Part model, mm, in its own coordinate system. Face numbers are marked on the shaded views. A direction names the side the tool comes from. Coordinates: 2 decimals unless noted, no trailing zeros. Order: outer loops, then holes, each group sorted by start corner. A loop starts at its lowest first (then second) coordinate and runs counter-clockwise, first axis right, second up.
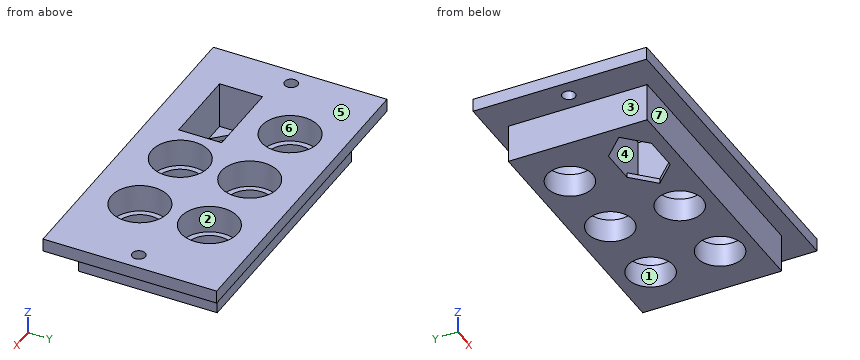
Autodesk Inventor part; units mm, degrees
ref_plane "YZ Plane" through (0, 0, 0) normal (1, 0, 0) x (0, 1, 0)
ref_plane "XZ Plane" through (0, 0, 0) normal (0, 1, 0) x (-1, 0, 0)
ref_plane "XY Plane" through (0, 0, 0) normal (0, 0, 1) x (1, 0, 0)
sketch "Sketch1" plane through (0, 0, 0) normal (0, 0, 1) x (1, 0, 0)
  line L0 (0, 0) -> (47.625, 0)
  line L1 (47.625, 0) -> (47.625, 25.4)
  line L2 (47.625, 25.4) -> (0, 25.4)
  line L3 (0, 25.4) -> (0, 0)
  circle A0 centre (38.1, 6.35) radius 5.207
  circle A1 centre (23.8125, 6.35) radius 5.207
  circle A2 centre (23.8125, 19.05) radius 5.207
  circle A3 centre (38.1, 19.05) radius 5.207
  circle A4 centre (9.525, 19.05) radius 5.207
  line L4 (2.2603, 10.287) -> (16.7383, 10.287)
  line L5 (16.7383, 10.287) -> (16.7383, 2.413)
  line L6 (16.7383, 2.413) -> (2.2603, 2.413)
  line L7 (2.2603, 2.413) -> (2.2603, 10.287)
  line L8 (-6.35, 28.575) -> (53.975, 28.575)
  line L9 (53.975, 28.575) -> (53.975, -3.175)
  line L10 (53.975, -3.175) -> (-6.35, -3.175)
  line L11 (-6.35, -3.175) -> (-6.35, 28.575)
  dimension "d0" = 47.625
  dimension "d1" = 25.4
  dimension "d2" = 10.414
  dimension "d3" = 10.414
  dimension "d4" = 10.414
  dimension "d5" = 10.414
  dimension "d6" = 10.414
  dimension "d9" = 14.478
  dimension "d10" = 7.874
  dimension "d27" = 60.325
  dimension "d28" = 31.75
extrude "Extrusion1" add sketch "Sketch1" against normal blind 9.398 contours L3 L2 L1 L0 | L8 L9 L10 L11
sketch "Sketch3" plane through (0, 0, -9.398) normal (0, 0, -1) x (-1, 0, 0)
  line L0 (6.35, 28.575) -> (-53.975, 28.575)
  line L1 (-53.975, 28.575) -> (-53.975, -3.175)
  line L2 (-53.975, -3.175) -> (6.35, -3.175)
  line L3 (6.35, -3.175) -> (6.35, 28.575)
  line L4 (-47.625, 25.4) -> (0, 25.4)
  line L5 (0, 25.4) -> (0, 0)
  line L6 (0, 0) -> (-47.625, 0)
  line L7 (-47.625, 0) -> (-47.625, 25.4)
extrude "Extrusion2" cut sketch "Sketch3" against normal blind 7.0104
sketch "Sketch4" plane through (0, 0, -9.398) normal (0, 0, -1) x (-1, 0, 0)
  circle A0 centre (-9.525, 19.05) radius 5.207
  circle A1 centre (-38.1, 19.05) radius 5.207
  circle A2 centre (-23.8125, 19.05) radius 5.207
  circle A3 centre (-23.8125, 6.35) radius 5.207
  circle A4 centre (-38.1, 6.35) radius 5.207
  circle A5 centre (-38.1, 19.05) radius 4.191
  circle A6 centre (-23.8125, 19.05) radius 4.191
  circle A7 centre (-9.525, 19.05) radius 4.191
  circle A8 centre (-38.1, 6.35) radius 4.191
  circle A9 centre (-23.8125, 6.35) radius 4.191
  dimension "d17" = 8.382
extrude "Extrusion3" add sketch "Sketch4" against normal blind 4.318
sketch "Sketch5" plane through (0, 0, -9.398) normal (0, 0, -1) x (-1, 0, 0)
  line L0 (-2.2603, 10.287) -> (-2.2603, 2.413)
  line L1 (-2.2603, 2.413) -> (-16.7383, 2.413)
  line L2 (-16.7383, 2.413) -> (-16.7383, 10.287)
  line L3 (-16.7383, 10.287) -> (-2.2603, 10.287)
  line L4 (-16.7383, 6.35) -> (-12.8013, 10.287)
  line L5 (-16.7383, 6.35) -> (-11.1705, 6.35) construction
  line L6 (-16.7383, 6.35) -> (-12.8013, 2.413)
  line L7 (-2.2603, 6.35) -> (-6.1973, 10.287)
  line L8 (-2.2603, 6.35) -> (-6.1973, 2.413)
  dimension "d20" = 45
extrude "Extrusion4" add sketch "Sketch5" against normal blind 0.889 contours L0 L7 L3 | L0 L1 L8 | L4 L2 L3 | L1 L2 L6
sketch "Sketch6" plane through (0, 0, 0) normal (0, 0, 1) x (1, 0, 0)
  circle A0 centre (-3.175, 12.7) radius 1.1938
  circle A1 centre (50.8, 12.7) radius 1.1938
  point P0 (0, 0)
  dimension "d23" = 2.3876
  dimension "d24" = 2.3876
extrude "Extrusion5" cut sketch "Sketch6" against normal blind 2.3876
properties part number "5 led mount idea"
(1) Pull direction Y, two halves, no side cores. Call the marked faces 4, 5, 6 and 7: +Y half, -Y half, draft (parallel to the pull), parting line (faces both ways), or undercut.
(2) Slice it at A-A, the plane z = -6.5. State how many separate pieces and enclosed holes the cut face has, then the cut area to 3 significant figures.
(3) Slice it at C-C, the plane x = 38.1. Give the cut face in (y, z) (3 decimals).
(4) Drop flat-ended pins along their axis: pin 1 (3.5 mm diameter, centred on x = 17, z = -5.5, fed in from -Y); pin 2 (1 mm diameter, centred on x = 31, z = -7.5, fed in from +Y); pin 3 (1 mm diameter, centred on y = 4, z = -7, fed in from +X) (3 decimals). Give the stop position or say it passes through.
(5) Probe line 1 (X direction, y = 6.35, z = -3.9) (1 decimal); line 2 (Y direction, x = 4, z = -1.5) (3 decimals); line 3 (Y direction, x = 26.5, z = -4). List the from-to ranges inside material, lowest first.
(6) Slice it at D-D, the plane x = 50.8. Give the cut face in (y, z) (3 decimals), then the cut area to 3 significant figures.
(7) Tool access for the marked faces 1, 2 and 3: list every direction of +Z, -Z, +X, -X, +Y, -Y with a clear straight run to the whole face (end or side of a thin tool).
Here are the results:
1. face 4: undercut
1. face 5: draft
1. face 6: undercut
1. face 7: -Y half
2. separate pieces: 1
2. enclosed holes: 6
2. area: 820 mm2
3. outline: (-3.175, -2.388) - (0, -2.388) - (0, -9.398) - (2.159, -9.398) - (2.159, -5.08) - (1.143, -5.08) - (1.143, 0) - (-3.175, 0) - close; (10.541, -9.398) - (14.859, -9.398) - (14.859, -5.08) - (13.843, -5.08) - (13.843, 0) - (11.557, 0) - (11.557, -5.08) - (10.541, -5.08) - close; (23.241, -9.398) - (25.4, -9.398) - (25.4, -2.388) - (28.575, -2.388) - (28.575, 0) - (24.257, 0) - (24.257, -5.08) - (23.241, -5.08) - close
4. pin 1: stops at y = 0
4. pin 2: stops at y = 25.4
4. pin 3: stops at x = 47.625
5. line 1: x = 0 to 2.3, 16.7 to 18.6, 29 to 32.9, 43.3 to 47.6
5. line 2: y = -3.175 to 2.413, 10.287 to 28.575
5. line 3: y = 0 to 1.89, 10.81 to 14.59, 23.51 to 25.4
6. outline: (-3.175, -2.388) - (11.506, -2.388) - (11.506, 0) - (-3.175, 0) - close; (13.894, -2.388) - (28.575, -2.388) - (28.575, 0) - (13.894, 0) - close
6. area: 70.1 mm2
7. face 1: +Z, -Z
7. face 2: +Z
7. face 3: -Z, -X, +Y, -Y
